The listing builds one solid part. Answer for the finished solid, in the listing's coordinates (mm). Give positions to 0.01 mm unless a question says otherwise; leave off trailing zeros. Write each loop counter-clockwise with the first axis right and the second up, starting at its lowest first coordinate (ties: lowest second). Pieces come first, ordered by that corner, then holes. Notation, with made-up numbers: (12.5, 78.25) - (70.5, 78.25) arc R22 ccw to (70.5, 105.25) - close; hole circle Ø6 at (61.25, -1.5). An arc over 180 degrees is marked (long way). One line per item, written item: value. Start each with the question number.
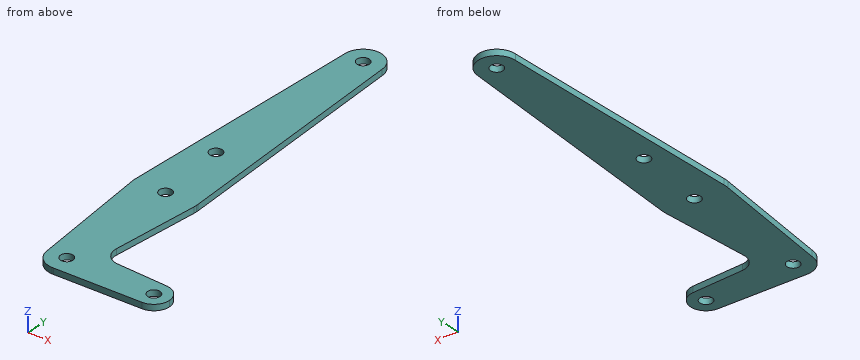
from build123d import *

# Parameters (mm, degrees)
F0_R     = 3.175
F1_DEPTH = 3.048


with BuildPart() as f1:
    # F0 (on Top) → F1 (new body)
    with BuildSketch(Plane.XY):
        with BuildLine():
            ThreePointArc((-9.525, 190.5), (0, 180.975), (9.525, 190.5))
            ThreePointArc((9.525, 190.5), (0, 200.025), (-9.525, 190.5))
        make_face()
        with Locations((0, 190.5)):
            Circle(F0_R, mode=Mode.SUBTRACT)
        with BuildLine():
            Line((15.855069, 64.295245), (9.525, 190.5))
            ThreePointArc((9.525, 190.5), (0, 180.975), (-9.525, 190.5))
            Line((-9.525, 190.5), (-15.855069, 64.295245))
            ThreePointArc((-15.855069, 64.295245), (0, 79.375), (15.855069, 64.295245))
        make_face()
        with Locations((-3.175, 99.886943)):
            Circle(F0_R, mode=Mode.SUBTRACT)
        with BuildLine():
            ThreePointArc((15.875, 63.5), (15.870016, 63.897747), (15.855069, 64.295245))
            ThreePointArc((15.855069, 64.295245), (0, 79.375), (-15.855069, 64.295245))
            ThreePointArc((-15.855069, 64.295245), (-15.869875, 63.096663), (-15.794203, 61.90038))
            ThreePointArc((-15.794203, 61.90038), (0, 47.625), (15.794203, 61.90038))
            ThreePointArc((15.794203, 61.90038), (15.854788, 62.699171), (15.875, 63.5))
        make_face()
        with Locations((0, 63.5)):
            Circle(F0_R, mode=Mode.SUBTRACT)
        with BuildLine():
            ThreePointArc((15.794203, 61.90038), (0, 47.625), (-15.794203, 61.90038))
            Line((-15.794203, 61.90038), (-9.525, 0))
            ThreePointArc((-9.525, 0), (0, 9.525), (9.525, 0))
            ThreePointArc((9.525, 0), (6.970557, -6.491299), (0.677344, -9.500886))
            Line((0.677344, -9.500886), (44.732405, -7.932475))
            ThreePointArc((44.732405, -7.932475), (36.5125, 0), (44.732405, 7.932475))
            Line((44.732405, 7.932475), (18.934103, 8.850924))
            ThreePointArc((18.934103, 8.850924), (13.224974, 11.57098), (11.307223, 17.59718))
            Line((11.307223, 17.59718), (15.794203, 61.90038))
        make_face()
        with BuildLine():
            ThreePointArc((9.525, 0), (0, 9.525), (-9.525, 0))
            ThreePointArc((-9.525, 0), (-6.735192, -6.735192), (0, -9.525))
            Line((0, -9.525), (0.677344, -9.500886))
            ThreePointArc((0.677344, -9.500886), (6.970557, -6.491299), (9.525, 0))
        make_face()
        Circle(F0_R, mode=Mode.SUBTRACT)
        with BuildLine():
            Line((0.677344, -9.500886), (0, -9.525))
            ThreePointArc((0, -9.525), (0.338886, -9.51897), (0.677344, -9.500886))
        make_face()
        with BuildLine():
            ThreePointArc((52.3875, 0), (50.161633, 5.51191), (44.732405, 7.932475))
            ThreePointArc((44.732405, 7.932475), (36.5125, 0), (44.732405, -7.932475))
            ThreePointArc((44.732405, -7.932475), (50.161633, -5.51191), (52.3875, 0))
        make_face()
        with Locations((44.45, 0)):
            Circle(F0_R, mode=Mode.SUBTRACT)
    extrude(amount=F1_DEPTH)


solid = f1.part
Item 1: Straight lines are drawn through the part: line 1 along X through (y, z) = (63, 1.5); line 2 along Y through (x, z) = (2, 2.95); line 3 along X through (y, z) = (190.5, 0.6) (3 decimals). For each, find the intervals that lie inside material, in ascending order.
Item 2: Find section B-B on x = 14. Determine the outline of the cut face in (y, z), plus the area to 3 significant figures.
Item 3: Find section A-A on z = 1.1. Give the number of separate pieces and of enclosed holes in the cut face, plus the area to 3 significant figures.
Item 4: Each of these flat-tipped pins is pushed along its axis until it touches: pin 1 Ø1.5 at (x, z) = (6.5, 1.5) entering from -Y; pin 2 Ø5.5 at (x, y) = (44.45, 0) entering from -Z; pin 3 Ø8.5 at (x, y) = (0, 63.5) entering from -Z; pin 4 Ø1 at (y, z) = (72.5, 1) entering from +X. Where does it stop, or does it pass through?
Item 5: Find section C-C on y = 49. Determine the outline of the cut face in (x, z).
Item 6: Find section D-D on x = -12. Determine the outline of the cut face in (y, z).
Values:
1. line 1: -15.87 to -3.14, 3.14 to 15.87
1. line 2: -9.45 to -2.47, 2.47 to 61.03, 65.97 to 188.03, 192.97 to 199.81
1. line 3: -9.525 to -3.175, 3.175 to 9.525
2. outline: (-9.03, 0) - (10.8, 0) - (10.8, 3.05) - (-9.03, 3.05) - close; (44.18, 0) - (101.28, 0) - (101.28, 3.05) - (44.18, 3.05) - close
2. area: 234 mm^2
3. separate pieces: 1
3. enclosed holes: 5
3. area: 5,700 mm^2
4. pin 1: y = -9.32
4. pin 2: through
4. pin 3: z = 0
4. pin 4: x = 15.47
5. outline: (-14.49, 0) - (14.49, 0) - (14.49, 3.05) - (-14.49, 3.05) - close
6. outline: (24.44, 0) - (141.16, 0) - (141.16, 3.05) - (24.44, 3.05) - close
